Geometry check sheet. Reference: the model listing, model coordinates, mm. A direction names the side the tool comes from. Give positions to 0.01 mm unless a question says otherwise; leave off trailing zeros. Write each loop counter-clockwise with the first axis right and the second up, starting at its lowest first coordinate (ties: lowest second). Pieces come first, ordered by that corner, then holes. Notation, with made-up numbers: (79.25, 85) -> (108.25, 85) arc R23 ccw to (108.25, 115) -> close; hole circle Ø1 at (62, 18.5). An arc over 180 degrees is marked (long way). One line per item, written item: value.
from build123d import *

# Parameters (mm, degrees)
F0_R     = 4.9
F1_DEPTH = 7


with BuildPart() as f1:
    # F0 (on Top) → F1 (new body)
    with BuildSketch(Plane.XY):
        with BuildLine():
            ThreePointArc((14.15, 0), (13.9757900194, -2.2135476803), (13.4574497056, -4.3725904704))
            ThreePointArc((13.4574497056, -4.3725904704), (12.400978844, -6.8145596858), (10.9060417797, -9.0155838801))
            Line((10.9060417797, -9.0155838801), (10.8695159641, -9.0820527185))
            Line((10.8695159641, -9.0820527185), (19.1268249694, -0.0593384625))
            Line((19.1268249694, -0.0593384625), (11.9964105728, 7.5310153528))
            Line((11.9964105728, 7.5310153528), (12.3111266381, 6.9755760265))
            ThreePointArc((12.3111266381, 6.9755760265), (13.6825608336, 3.6069417844), (14.15, 0))
        make_face()
        with BuildLine():
            Line((10.8695159641, -9.0820527185), (10.4385144096, -9.5530056485))
            ThreePointArc((10.4385144096, -9.5530056485), (5.702958446, -12.9498557893), (0, -14.15))
            ThreePointArc((0, -14.15), (-2.6489181852, -13.8998464901), (-5.2041775461, -13.1582307347))
            Line((-5.2041775461, -13.1582307347), (-5.2786802657, -13.1440326205))
            Line((-5.2786802657, -13.1440326205), (5.8540797326, -18.2090281165))
            Line((5.8540797326, -18.2090281165), (10.8695159641, -9.0820527185))
        make_face()
        with BuildLine():
            Line((19.1268249694, -0.0593384625), (10.8695159641, -9.0820527185))
            Line((10.8695159641, -9.0820527185), (5.8540797326, -18.2090281165))
            Line((5.8540797326, -18.2090281165), (21.2854911766, -25.2297515915))
            ThreePointArc((21.2854911766, -25.2297515915), (19.5794245005, -14.1382025948), (30.685746847, -12.531116229))
            Line((30.685746847, -12.531116229), (30.6560666179, -12.3322609697))
            Line((30.6560666179, -12.3322609697), (19.1268249694, -0.0593384625))
        make_face()
        with BuildLine():
            ThreePointArc((8.3171613199, 11.4475904704), (10.3131446045, 9.6882169859), (11.9444820487, 7.5862934684))
            Line((11.9444820487, 7.5862934684), (11.9964105728, 7.5310153528))
            Line((11.9964105728, 7.5310153528), (5.9669481954, 18.1723549299))
            Line((5.9669481954, 18.1723549299), (-3.4553264872, 13.7364761763))
            Line((-3.4553264872, 13.7364761763), (-2.8298212171, 13.8641484369))
            ThreePointArc((-2.8298212171, 13.8641484369), (2.9979432037, 13.8287684393), (8.3171613199, 11.4475904704))
        make_face()
        with BuildLine():
            Line((5.9669481954, 18.1723549299), (11.9964105728, 7.5310153528))
            Line((11.9964105728, 7.5310153528), (19.1268249694, -0.0593384625))
            Line((19.1268249694, -0.0593384625), (30.5724981628, 12.4472830804))
            ThreePointArc((30.5724981628, 12.4472830804), (19.4966046172, 14.2521943848), (21.4002170069, 25.311551623))
            Line((21.4002170069, 25.311551623), (21.2019227215, 25.3447737022))
            Line((21.2019227215, 25.3447737022), (5.9669481954, 18.1723549299))
        make_face()
        with BuildLine():
            Line((-2.2554315903, -32.9665301396), (5.8540797326, -18.2090281165))
            Line((5.8540797326, -18.2090281165), (-5.2786802657, -13.1440326205))
            Line((-5.2786802657, -13.1440326205), (-15.5088047218, -11.1944598156))
            Line((-15.5088047218, -11.1944598156), (-17.4173411484, -28.0401270917))
            ThreePointArc((-17.4173411484, -28.0401270917), (-8.6681623959, -22.6786234566), (-2.0039946697, -30.4813613473))
            ThreePointArc((-2.0039946697, -30.4813613473), (-2.1125879849, -31.7867279132), (-2.4353824853, -33.0562073695))
            Line((-2.4353824853, -33.0562073695), (-2.2554315903, -32.9665301396))
        make_face()
        with BuildLine():
            Line((-3.4553264872, 13.7364761763), (5.9669481954, 18.1723549299))
            Line((5.9669481954, 18.1723549299), (-2.390648191, 32.9225956028))
            ThreePointArc((-2.390648191, 32.9225956028), (-2.101256779, 31.7171936211), (-2.0039946697, 30.4813613473))
            ThreePointArc((-2.0039946697, 30.4813613473), (-8.7377949727, 22.6679127958), (-17.4596853701, 28.17451544))
            Line((-17.4596853701, 28.17451544), (-17.5525577492, 27.9961925549))
            Line((-17.5525577492, 27.9961925549), (-15.4390481756, 11.2904714648))
            Line((-15.4390481756, 11.2904714648), (-3.4553264872, 13.7364761763))
        make_face()
        with BuildLine():
            Line((32.3202289253, -23.4820208291), (21.2854911766, -25.2297515915))
            ThreePointArc((21.2854911766, -25.2297515915), (27.1648269435, -26.6412552267), (32.3202289253, -23.4820208291))
        make_face()
        with BuildLine():
            ThreePointArc((30.685746847, -12.531116229), (19.5794245005, -14.1382025948), (21.2854911766, -25.2297515915))
            Line((21.2854911766, -25.2297515915), (32.3202289253, -23.4820208291))
            Line((32.3202289253, -23.4820208291), (30.685746847, -12.531116229))
        make_face()
        with Locations((25.9289946697, -18.838517336)):
            Circle(F0_R, mode=Mode.SUBTRACT)
        with BuildLine():
            Line((-15.5088047218, -11.1944598156), (-5.2786802657, -13.1440326205))
            Line((-5.2786802657, -13.1440326205), (-5.8597700568, -12.8796581819))
            ThreePointArc((-5.8597700568, -12.8796581819), (-10.5537337042, -9.4255612513), (-13.4574497056, -4.3725904704))
            ThreePointArc((-13.4574497056, -4.3725904704), (-14.0381003158, -1.7760178835), (-14.1224003867, 0.8833500542))
            Line((-14.1224003867, 0.8833500542), (-14.1319197841, 0.9585938098))
            Line((-14.1319197841, 0.9585938098), (-15.5088047218, -11.1944598156))
        make_face()
        with BuildLine():
            Line((32.3202289253, 23.4820208291), (30.5724981628, 12.4472830804))
            ThreePointArc((30.5724981628, 12.4472830804), (32.9679462108, 15.251992388), (33.8289946697, 18.838517336))
            ThreePointArc((33.8289946697, 18.838517336), (33.4423411484, 21.2797515915), (32.3202289253, 23.4820208291))
        make_face()
        with BuildLine():
            ThreePointArc((21.4002170069, 25.311551623), (19.4966046172, 14.2521943848), (30.5724981628, 12.4472830804))
            Line((30.5724981628, 12.4472830804), (32.3202289253, 23.4820208291))
            Line((32.3202289253, 23.4820208291), (21.4002170069, 25.311551623))
        make_face()
        with Locations((25.9289946697, 18.838517336)):
            Circle(F0_R, mode=Mode.SUBTRACT)
        with BuildLine():
            Line((-3.5239458956, 13.7041710922), (-3.4553264872, 13.7364761763))
            Line((-3.4553264872, 13.7364761763), (-15.4390481756, 11.2904714648))
            Line((-15.4390481756, 11.2904714648), (-14.1319197841, 0.9585938098))
            Line((-14.1319197841, 0.9585938098), (-14.0600515027, 1.5929380844))
            ThreePointArc((-14.0600515027, 1.5929380844), (-12.2255248084, 7.1245381015), (-8.3171613199, 11.4475904704))
            ThreePointArc((-8.3171613199, 11.4475904704), (-6.0271049475, 12.8022070735), (-3.5239458956, 13.7041710922))
        make_face()
        with BuildLine():
            Line((-12.3452289253, 37.994707826), (-2.390648191, 32.9225956028))
            ThreePointArc((-2.390648191, 32.9225956028), (-6.3174697218, 37.5203128883), (-12.3452289253, 37.994707826))
        make_face()
        with BuildLine():
            ThreePointArc((-2.0039946697, 30.4813613473), (-2.101256779, 31.7171936211), (-2.390648191, 32.9225956028))
            Line((-2.390648191, 32.9225956028), (-12.3452289253, 37.994707826))
            Line((-12.3452289253, 37.994707826), (-17.4596853701, 28.17451544))
            ThreePointArc((-17.4596853701, 28.17451544), (-8.7377949727, 22.6679127958), (-2.0039946697, 30.4813613473))
        make_face()
        with Locations((-9.9039946697, 30.4813613473)):
            Circle(F0_R, mode=Mode.SUBTRACT)
        with BuildLine():
            Line((-12.3452289253, -37.994707826), (-2.4353824853, -33.0562073695))
            ThreePointArc((-2.4353824853, -33.0562073695), (-2.1125879849, -31.7867279132), (-2.0039946697, -30.4813613473))
            ThreePointArc((-2.0039946697, -30.4813613473), (-8.6681623959, -22.6786234566), (-17.4173411484, -28.0401270917))
            Line((-17.4173411484, -28.0401270917), (-12.3452289253, -37.994707826))
        make_face()
        with Locations((-9.9039946697, -30.4813613473)):
            Circle(F0_R, mode=Mode.SUBTRACT)
        with BuildLine():
            ThreePointArc((-12.3452289253, -37.994707826), (-6.3803844615, -37.5520169817), (-2.4353824853, -33.0562073695))
            Line((-2.4353824853, -33.0562073695), (-12.3452289253, -37.994707826))
        make_face()
        with BuildLine():
            Line((30.685746847, -12.531116229), (32.3202289253, -23.4820208291))
            ThreePointArc((32.3202289253, -23.4820208291), (33.4423411484, -21.2797515915), (33.8289946697, -18.838517336))
            ThreePointArc((33.8289946697, -18.838517336), (32.9996503041, -15.3149071277), (30.685746847, -12.531116229))
        make_face()
        with BuildLine():
            Line((-32.05, -8.0421751477), (-15.5088047218, -11.1944598156))
            Line((-15.5088047218, -11.1944598156), (-14.1319197841, 0.9585938098))
            Line((-14.1319197841, 0.9585938098), (-15.4390481756, 11.2904714648))
            Line((-15.4390481756, 11.2904714648), (-32.05, 7.9))
            ThreePointArc((-32.05, 7.9), (-26.4638564286, 5.5861435714), (-24.15, 0))
            ThreePointArc((-24.15, 0), (-26.5138947982, -5.6357376797), (-32.1908959985, -7.8987434645))
            Line((-32.1908959985, -7.8987434645), (-32.05, -8.0421751477))
        make_face()
        with BuildLine():
            ThreePointArc((32.3202289253, 23.4820208291), (27.2343612356, 26.6299240208), (21.4002170069, 25.311551623))
            Line((21.4002170069, 25.311551623), (32.3202289253, 23.4820208291))
        make_face()
        with BuildLine():
            Line((-17.4596853701, 28.17451544), (-12.3452289253, 37.994707826))
            ThreePointArc((-12.3452289253, 37.994707826), (-16.9106823157, 34.1305158016), (-17.4596853701, 28.17451544))
        make_face()
        with BuildLine():
            ThreePointArc((-17.4173411484, -28.0401270917), (-16.9429462108, -34.0678862952), (-12.3452289253, -37.994707826))
            Line((-12.3452289253, -37.994707826), (-17.4173411484, -28.0401270917))
        make_face()
        with BuildLine():
            Line((-39.95, 0), (-32.05, 7.9))
            ThreePointArc((-32.05, 7.9), (-37.6361435714, 5.5861435714), (-39.95, 0))
        make_face()
        with BuildLine():
            ThreePointArc((-24.15, 0), (-26.4638564286, 5.5861435714), (-32.05, 7.9))
            Line((-32.05, 7.9), (-39.95, 0))
            Line((-39.95, 0), (-32.1908959985, -7.8987434645))
            ThreePointArc((-32.1908959985, -7.8987434645), (-26.5138947982, -5.6357376797), (-24.15, 0))
        make_face()
        with Locations((-32.05, 0)):
            Circle(F0_R, mode=Mode.SUBTRACT)
        with BuildLine():
            ThreePointArc((-39.95, 0), (-37.6857376797, -5.5361052018), (-32.1908959985, -7.8987434645))
            Line((-32.1908959985, -7.8987434645), (-39.95, 0))
        make_face()
    extrude(amount=F1_DEPTH)


solid = f1.part
1) Tool access check on faces 1 (the flat face through (-16.51, 19.76, 3.45)), 2 (the flat face through (13.69, 21.81, 3.45)), 3 (the cylindrical face through (5.42, 13.07, 3.45)), 4 (the flat face through (24.77, 6.106, 3.451)), 5 (the flat face through (1.743, -25.691, 3.451)). Record the directions out of +Z, -Z, +X, -X, +Y, -Y that give a thin tool (end or side, any length) a straight path to the whole face; none if there is none.
Verdict:
face 1: +Z, -Z, -X
face 2: +Z, -Z, +Y
face 3: +Z, -Z
face 4: +Z, -Z, +X
face 5: +Z, -Z, -Y
2) Sectioned sample at B-B on x = -30. Record the cut outline in (y, z), plus the area to 3 significant figures.
Verdict:
outline: (-8.43, 0) -> (-4.45, 0) -> (-4.45, 7) -> (-8.43, 7) -> close; (4.45, 0) -> (8.32, 0) -> (8.32, 7) -> (4.45, 7) -> close
area: 55.0 mm^2
3) Mould release check, pull along X, two halves, no side actions. Record for faces 6 (the flat face through (-16.45, -19.5, 3.45)), 7 (the cylindrical face through (30.455, -20.715, 3.451)), 8 (the flat face through (24.97, -6.28, 3.45)): released by +X, released by -X, zero draft, split by the parting line, or undercut.
Verdict:
face 6: released by -X
face 7: undercut
face 8: released by +X
4) Depth check by flat-ended pin: pin 1 Ø2 at (x, z) = (20, 2) entering from -Y; pin 2 Ø3 at (y, z) = (-5.5, 1.5) entering from -X; pin 3 Ø12.5 at (x, y) = (25.93, 18.84) entering from +Z; pin 4 Ø1 at (x, z) = (-8, 5.5) entering from -Y. Enter the tip coordinate at first touch or a pass-through.
Verdict:
pin 1: y = -25.1
pin 2: x = -38.86
pin 3: z = 7
pin 4: y = -38.26
5) Sectioned sample at C-C on y = -2.5. Record the cut outline in (x, z), plus the area to 3 significant figures.
Verdict:
outline: (-39.54, 0) -> (-36.26, 0) -> (-36.26, 7) -> (-39.54, 7) -> close; (-27.84, 0) -> (-13.93, 0) -> (-13.93, 7) -> (-27.84, 7) -> close; (13.93, 0) -> (21.42, 0) -> (21.42, 7) -> (13.93, 7) -> close
area: 173 mm^2
6) Sectioned sample at D-D on z = 3.25. Give the number of separate pieces and of enclosed holes in the cut face, plus the area to 3 significant figures.
Verdict:
separate pieces: 1
enclosed holes: 6
area: 1,950 mm^2
7) Scan lines: probe 1 along Y at (x, z) = (-32.05, 2.5); probe 2 along Y at (x, z) = (-10.5, 1); probe 3 along Y at (x, z) = (25, 6.75). Record each from-to range of solid material in increasing order.
Verdict:
probe 1: -8.04 to -4.9, 4.9 to 7.9
probe 2: -38.36 to -35.34, -25.62 to -9.49, 9.49 to 25.62, 35.34 to 38.36
probe 3: -26.68 to -23.65, -14.03 to -6.31, 6.36 to 14.03, 23.65 to 26.68
8) Sectioned sample at A-A on y = 9. Record the cut outline in (x, z), plus the area to 3 significant figures.
Verdict:
outline: (-26.66, 0) -> (-10.92, 0) -> (-10.92, 7) -> (-26.66, 7) -> close; (10.92, 0) -> (27.42, 0) -> (27.42, 7) -> (10.92, 7) -> close
area: 226 mm^2
